Geometry: final body of the model. Coordinates: model frame, mm. Face numbers are marked on the shaded views. A direction names the side the tool comes from. Coordinates: 2 decimals unless noted, no trailing zeros. Write each loop counter-clockwise with the first axis right and the second up, starting at its lowest first coordinate (ties: lowest second). Pieces come first, ordered by that corner, then holes. Notation, with made-up numbers: (7, 17.25) - (63, 17.25) arc R6 ccw to (63, 28.25) - close; hole circle Ø9 at (23.25, 70). An arc over 180 degrees is marked (long way). Answer as a JSON object with one key per item and string values. Group by question number.
Item 1: Mould query, pull axis X, two halves, no side actions, for the marked faces 1, 2, 3 and 4. Classes: pulls with the +X half, pulls with the -X half, needs draft (parallel to the pull), parting line crosses it, or undercut.
Item 2: Line query: line 1 along X through (y, z) = (2.5, 0) (3 decimals); line 2 along X through (y, z) = (6, 0) (3 decimals); line 3 along Z through (x, y) = (10, 8.5). Output: solid intervals per line, ascending. Write a range as from..to.
Item 3: Section B-B on y = 5. State how many separate pieces and enclosed holes the cut face has, and give its area (3 significant figures).
Item 4: Section D-D on x = -50. Return loops of the section in (y, z), and give its area (3 significant figures).
Item 5: Section A-A on z = 0. Return loops of the section in (x, y) (3 decimals), and give its area (3 significant figures).
Item 6: First-contact query: pin 1 Ø8 at (x, z) = (43, -7) entering from -Y; pin 2 Ø10 at (x, z) = (44.5, -33) entering from +Y; pin 3 Ø3 at (x, y) = (-24.5, 14) entering from -Z; pin 4 Ø6 at (y, z) = (10.5, 36) entering from +X. Flat tips, straight axial feed; report the tip coordinate or a pass-through.
Item 7: Set-up query: the marked faces 5 and 6. Return all of +Z, -Z, +X, -X, +Y, -Y with unobstructed straight access to the full face (end or side cutting, diameter ignored); none if empty.
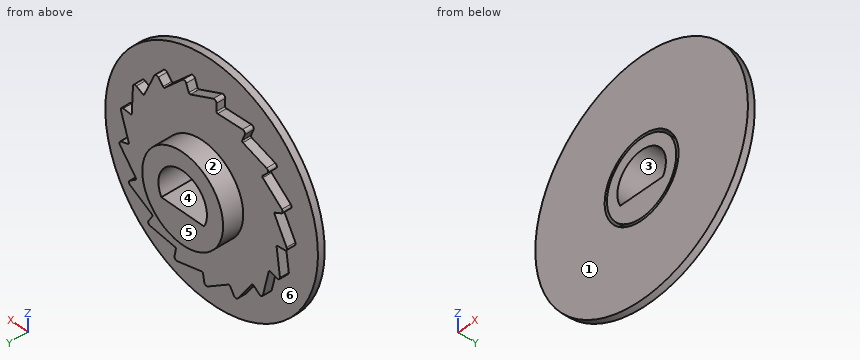
```python
from build123d import *

# Parameters (mm, degrees)
SKETCH1_R           = 58.42
BOSS_EXTRUDE1_DEPTH = 3.429
SKETCH2_R           = 47.700633093
BOSS_EXTRUDE3_DEPTH = 4.445
CUT_EXTRUDE2_START  = -4.445
CUT_EXTRUDE2_DEPTH  = 4.445
CIRPATTERN1_COUNT   = 17
FILLET1_R           = 1.27
FILLET2_R           = 0.635
SKETCH5_R           = 22.225
BOSS_EXTRUDE4_DEPTH = 10.16
CUT_EXTRUDE3_DEPTH  = 85.563691712
SKETCH7_R           = 20.32
SKETCH7_R_2         = 19.05
CUT_EXTRUDE4_DEPTH  = 10.16


with BuildPart() as part:
    # Sketch1 → Boss-Extrude1 (new body)
    with BuildSketch(Plane(origin=(0, 0, 0), x_dir=(1, 0, 0), z_dir=(0, 1, 0))):
        with Locations(Location((0, 0, 0), (0, 0, 270))):
            Circle(SKETCH1_R)
    extrude(amount=BOSS_EXTRUDE1_DEPTH)

    # Sketch2 → Boss-Extrude3 (add)
    with BuildSketch(Plane(origin=(0, 3.429, 0), x_dir=(1, 0, 0), z_dir=(0, 1, 0))):
        with Locations(Location((0, 0, 0), (0, 0, 270))):
            Circle(SKETCH2_R)
    extrude(amount=BOSS_EXTRUDE3_DEPTH)

    # Sketch4 → Cut-Extrude2 (cut)
    with BuildSketch(Plane(origin=(0, 7.874, 0), x_dir=(1, 0, 0), z_dir=(0, 1, 0)).offset(CUT_EXTRUDE2_START)):
        with BuildLine():
            Line((-1.27, 47.683723612), (0, 40.64))
            Line((0, 40.64), (17.007917051, 44.565470435))
            ThreePointArc((17.007917051, 44.565470435), (8.021931438, 47.021261292), (-1.27, 47.683723612))
        make_face()
    cut_extrude2 = extrude(amount=CUT_EXTRUDE2_DEPTH, mode=Mode.SUBTRACT)

    # CirPattern1: Cut-Extrude2 ×17 about axis
    cirpattern1_axis = Axis((0, 0, 0), (0, 1, 0))
    for i in range(1, CIRPATTERN1_COUNT):
        add(cut_extrude2.rotate(cirpattern1_axis, i * 360 / CIRPATTERN1_COUNT), mode=Mode.SUBTRACT)

    # Fillet1
    fillet1_edges = [part.edges().sort_by_distance(p)[0] for p in [
        (-1.160233877, 5.6515, -47.07493445),
        (15.923541887, 5.6515, -44.315193895),
        (-18.087313626, 5.6515, -43.476944257),
        (-32.571601445, 5.6515, -34.007151828),
        (-42.656914003, 5.6515, -19.944505104),
        (-46.981173955, 5.6515, -3.18824245),
        (-44.960366033, 5.6515, 13.998610014),
        (-36.867411544, 5.6515, 29.294872626),
        (-23.795308837, 5.6515, 40.634700362),
        (-7.509517816, 5.6515, 46.486586649),
        (9.790475196, 5.6515, 46.060201819),
        (25.768210283, 5.6515, 39.413131504),
        (38.265805785, 5.6515, 27.443099384),
        (45.595392177, 5.6515, 11.766724625),
        (46.767068202, 5.6515, -5.498811497),
        (41.622592522, 5.6515, -22.021702656),
        (30.856755083, 5.6515, -35.570440844),
    ]]
    fillet(fillet1_edges, radius=FILLET1_R)

    # Fillet2
    fillet2_edges = [part.edges().sort_by_distance(p)[0] for p in [
        (0, 5.6515, -40.64),
        (14.680861314, 5.6515, -37.895671403),
        (-14.680861314, 5.6515, -37.895671403),
        (-27.378990958, 5.6515, -30.033322396),
        (-36.379436161, 5.6515, -18.114806779),
        (-40.466636925, 5.6515, -3.749786129),
        (-39.088594139, 5.6515, 11.121663917),
        (-32.431420117, 5.6515, 24.491071622),
        (-21.394203099, 5.6515, 34.552824396),
        (-7.467580404, 5.6515, 39.948026771),
        (7.467580404, 5.6515, 39.948026771),
        (21.394203099, 5.6515, 34.552824396),
        (32.431420117, 5.6515, 24.491071622),
        (39.088594139, 5.6515, 11.121663917),
        (40.466636925, 5.6515, -3.749786129),
        (36.379436161, 5.6515, -18.114806779),
        (27.378990958, 5.6515, -30.033322396),
    ]]
    fillet(fillet2_edges, radius=FILLET2_R)

    # Sketch5 → Boss-Extrude4 (add)
    with BuildSketch(Plane(origin=(0, 7.874, 0), x_dir=(1, 0, 0), z_dir=(0, 1, 0))):
        with Locations(Location((0, 0, 0), (0, 0, 270))):
            Circle(SKETCH5_R)
    extrude(amount=BOSS_EXTRUDE4_DEPTH)

    # Sketch6 → Cut-Extrude3 (cut, through all)
    with BuildSketch(Plane(origin=(0, 18.034, 0), x_dir=(1, 0, 0), z_dir=(0, 1, 0))):
        with BuildLine():
            Line((-11.7475, 6.310187695), (11.7475, 6.310187695))
            ThreePointArc((11.7475, 6.310187695), (0, -13.335), (-11.7475, 6.310187695))
        make_face()
    extrude(amount=-CUT_EXTRUDE3_DEPTH, mode=Mode.SUBTRACT)

    # Sketch7 → Cut-Extrude4 (cut)
    with BuildSketch(Plane.XZ):
        with Locations(Location((0, 0, 0), (0, 0, 270))):
            Circle(SKETCH7_R)
        with Locations(Location((0, 0, 0), (0, 0, 270))):
            Circle(SKETCH7_R_2, mode=Mode.SUBTRACT)
    extrude(amount=-CUT_EXTRUDE4_DEPTH, mode=Mode.SUBTRACT)


solid = part.part
```
Checks:
{
 "1": {"face 1": "needs draft", "face 2": "parting line crosses it", "face 3": "undercut", "face 4": "undercut"},
 "2": {"line 1": "-58.42..-20.32, -19.05..-13.335, 13.335..19.05, 20.32..58.42", "line 2": "-45.223..-20.32, -19.05..-13.335, 13.335..19.05, 20.32..41.706", "line 3": "-19.85..-17.69, -16.21..-6.31, 8.82..16.21, 17.69..19.85"},
 "3": {"separate pieces": "2", "enclosed holes": "2", "area": "5,290 mm^2"},
 "4": {"outline": "(0, -30.21) - (3.43, -30.21) - (3.43, 30.21) - (0, 30.21) - close", "area": "207 mm^2"},
 "5": {"outline": "(-58.42, 0) - (-20.32, 0) - (-20.32, 10.16) - (-19.05, 10.16) - (-19.05, 0) - (-13.335, 0) - (-13.335, 18.034) - (-22.225, 18.034) - (-22.225, 7.874) - (-45.223, 7.874) - (-45.223, 3.429) - (-58.42, 3.429) - close; (13.335, 0) - (19.05, 0) - (19.05, 10.16) - (20.32, 10.16) - (20.32, 0) - (58.42, 0) - (58.42, 3.429) - (41.706, 3.429) - (41.706, 7.874) - (22.225, 7.874) - (22.225, 18.034) - (13.335, 18.034) - close", "area": "732 mm^2"},
 "6": {"pin 1": "y = 0", "pin 2": "y = 3.43", "pin 3": "through", "pin 4": "x = 27.94"},
 "7": {"face 5": "+Z, -Z, +X, -X, +Y", "face 6": "+Y"}
}
